Design review of the part built by this model. Coordinates are the model's own, in mm. A direction names the side the tool comes from. Give positions to 0.01 mm unless a question says otherwise; leave off trailing zeros. Loops run counter-clockwise (first coordinate to the right, second up) from the corner with the lowest first, then second, coordinate; pieces in that order, holes last. Notation, with made-up numbers: (54, 62) - (89, 62) arc R18 cw to (89, 68) - close; hole circle Ø3 at (-14.75, -25). An arc over 180 degrees is marked (long way). Write each question's results on one line, items separated by ' | '.
from build123d import *

# Parameters (mm, degrees)
SKETCH_R          = 2.5
PAD_DEPTH         = 4
SKETCH001_R       = 5
SKETCH001_R_2     = 2.5
PAD001_DEPTH      = 7
FILLET_R          = 5
SKETCH002_W       = 12.9
SKETCH002_H       = 8.550953
POCKET_DEPTH      = 38.001
POCKET_DEPTH_BACK = 5.001


with BuildPart() as part:
    # Sketch → Pad (new body)
    with BuildSketch(Plane.XY):
        with BuildLine():
            Line((-10, -5), (10, -5))
            ThreePointArc((10, -5), (15, 0.000362), (9.999276, 5))
            Line((7.5, 5), (9.999276, 5))
            Line((7.5, 38), (7.5, 5))
            Line((-7.5, 38), (7.5, 38))
            Line((-7.5, 38), (-7.5, 5))
            Line((-7.5, 5), (-9.999276, 5))
            ThreePointArc((-9.999276, 5), (-15, 0.000362), (-10, -5))
        make_face()
        with Locations((-10, 0)):
            Circle(SKETCH_R, mode=Mode.SUBTRACT)
        with Locations((10, 0)):
            Circle(SKETCH_R, mode=Mode.SUBTRACT)
        with BuildLine():
            ThreePointArc((2.5, 33), (0, 35.5), (-2.5, 33))
            Line((-2.5, 33), (-2.5, 0))
            ThreePointArc((-2.5, 0), (0, -2.5), (2.5, 0))
            Line((2.5, 33), (2.5, 0))
        make_face(mode=Mode.SUBTRACT)
    extrude(amount=PAD_DEPTH)

    # Sketch001 (on Face16 of Pad) → Pad001 (join)
    with BuildSketch(Plane.XY.offset(4)):
        with Locations((10, 0)):
            Circle(SKETCH001_R)
        with Locations((10, 0)):
            Circle(SKETCH001_R_2, mode=Mode.SUBTRACT)
        with Locations((-10, 0)):
            Circle(SKETCH001_R)
        with Locations((-10, 0)):
            Circle(SKETCH001_R_2, mode=Mode.SUBTRACT)
    extrude(amount=PAD001_DEPTH)

    # Fillet
    fillet_edges = [part.edges().sort_by_distance(p)[0] for p in [
        (-7.5, 38, 2),
        (7.5, 38, 2),
    ]]
    fillet(fillet_edges, radius=FILLET_R)

    # Sketch002 → Pocket (cut, two sides)
    with BuildSketch(Plane.XZ) as pocket_sk:
        with Locations((0, 8.275476)):
            Rectangle(SKETCH002_W, SKETCH002_H)
    extrude(amount=-POCKET_DEPTH, mode=Mode.SUBTRACT)
    extrude(pocket_sk.sketch, amount=POCKET_DEPTH_BACK, mode=Mode.SUBTRACT)


solid = part.part
(1) Take a section at A-A on y = 20.5. Give the boundary of the cut face in (x, z), plus the area to 3 significant figures.
Answers below:
outline: (-7.5, 0) - (-2.5, 0) - (-2.5, 4) - (-7.5, 4) - close; (2.5, 0) - (7.5, 0) - (7.5, 4) - (2.5, 4) - close | area: 40.0 mm2
(2) Take a section at D-D on y = 2. Give the boundary of the cut face in (x, z).
Answers below:
outline: (-14.58, 0) - (-11.5, 0) - (-11.5, 11) - (-14.58, 11) - close; (-8.5, 0) - (-2.5, 0) - (-2.5, 4) - (-6.45, 4) - (-6.45, 11) - (-8.5, 11) - close; (2.5, 0) - (8.5, 0) - (8.5, 11) - (6.45, 11) - (6.45, 4) - (2.5, 4) - close; (11.5, 0) - (14.58, 0) - (14.58, 11) - (11.5, 11) - close
(3) Tool access review of faces 5 (the flat face through (-6.45, 0, 7)), 6 (the flat face through (7.3, -4.5, 4)), 7 (the flat face through (-7.5, 19, 2)): name each direction out of +Z, -Z, +X, -X, +Y, -Y from which nothing blocks a thin tool from reaching the whole face with its end or side.
Answers below:
face 5: +Z, +Y, -Y | face 6: +Z, -Y | face 7: +Z, -Z, -X, +Y
(4) Draft analysis for pull direction Y (two halves, no side actions). For faces 1 (the cylindrical face through (-15, 0, 5)), 2 (the flat face through (0, 38, 2)), 3 (the cylindrical face through (-0.1, -2.5, 2)), 4 (the flat face through (-13, 0, 11)), state which applies: pulls with the +Y half, pulls with the -Y half, needs draft (parallel to the pull), parting line crosses it, or undercut.
Answers below:
face 1: parting line crosses it | face 2: pulls with the +Y half | face 3: undercut | face 4: needs draft
(5) Wall thickness on line 1 along Y through (x, z) = (-10, 3.25); line 2 along X through (y, z) = (27.5, 1.25); line 3 along Z through (x, y) = (3.5, 10.5): over which ranges is each line inside the solid? List them lowest first. Write a range as from..to.
Answers below:
line 1: -5..-2.5, 2.5..5 | line 2: -7.5..-2.5, 2.5..7.5 | line 3: 0..4
(6) Take a section at B-B on z = 6.5. Give the boundary of the cut face in (x, y), plus the area to 3 significant figures.
Answers below:
outline: (-6.45, -3.52) - (-6.45, 3.52) arc R5 ccw (long way) to start; (6.45, -3.52) arc R5 ccw (long way) to (6.45, 3.52) - close; hole circle Ø5 at (-10, 0); hole circle Ø5 at (10, 0) | area: 104 mm2
(7) Take a section at C-C on x = 0. Give the boundary of the cut face in (y, z).
Answers below:
outline: (-5, 0) - (-2.5, 0) - (-2.5, 4) - (-5, 4) - close; (35.5, 0) - (38, 0) - (38, 4) - (35.5, 4) - close
(8) Insertion check: P1, Ø3, axis at x = -7, z = 6.5, coming from the +Y side; P2, Ø2.5, axis at x = 9, z = 3, coming from the +Y side; P3, Ø3, axis at x = -8.5, y = 16, coming from the +Z side; P4, Ø4, axis at x = -3.5, z = 9, coming from the -Y side. Each pin has a flat end and moves straight along its axis. Give the tip position at first contact, or say it passes through.
Answers below:
P1: y = 4.77 | P2: y = 5 | P3: z = 4 | P4: through
